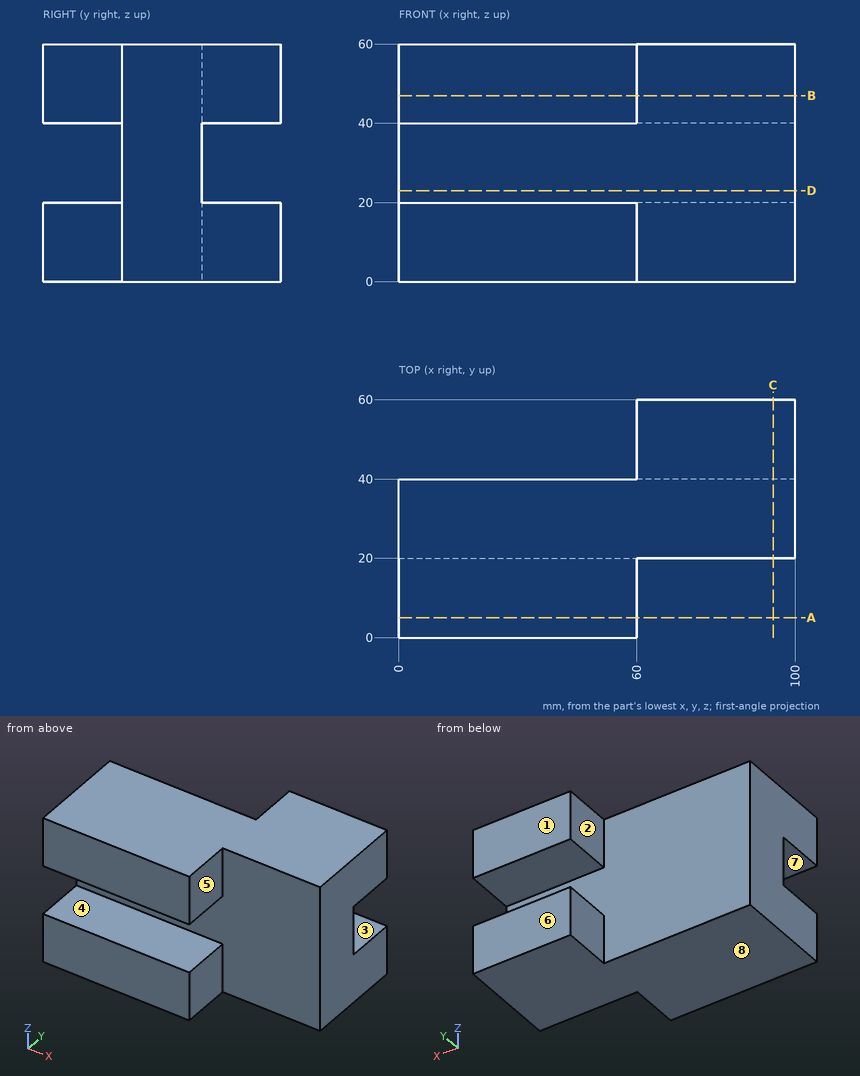
Input: dimensioned drawing with shaded views. Units: mm. Origin: part minimum x, y, z. A direction names the side the tool comes from. Coordinates: 2 decimals unless noted, no trailing zeros. Order: outer loops, then holes, each group sorted by start corner. A loop starts at its lowest first (then second) coordinate and runs counter-clockwise, first axis right, second up.
Item 1: Section query D-D (z = 23). Output: boundary loops of the cut face in (x, y), then the cut area to 3 significant figures.
Answer:
outline: (0, 20) - (100, 20) - (100, 40) - (0, 40) - close
area: 2,000 mm2
Item 2: Section query A-A (y = 5). Output: boundary loops of the cut face in (x, z).
Answer:
outline: (0, 0) - (60, 0) - (60, 20) - (0, 20) - close; (0, 40) - (60, 40) - (60, 60) - (0, 60) - close
Item 3: Material intervals for line 1 along Z through (x, y) = (78, 42.5); line 2 along X through (y, z) = (46.5, 5.5); line 3 along Y through (x, z) = (94.5, 53), sorted ascending.
Answer:
line 1: z = 0 to 20, 40 to 60
line 2: x = 60 to 100
line 3: y = 20 to 60
Item 4: Contact query for flat-ended pins moving along their axis: P1, Ø10, axis at x = 32, z = 25.5, coming from the -Y side; P2, Ø16, axis at y = 8, z = 14, coming from the +X side; P3, Ø6, axis at y = 48, z = 10.5, coming from the -X side. Output: stop coordinate, or through.
Answer:
P1: stops at y = 20
P2: stops at x = 60
P3: stops at x = 60
Item 5: Draft query along Z for the marked faces 6, 7 and 8. Return one class per face: released by +Z, released by -Z, zero draft, split by the parting line, or undercut.
Answer:
face 6: zero draft
face 7: undercut
face 8: released by -Z
Item 6: Section query B-B (z = 47). Output: boundary loops of the cut face in (x, y), then the cut area to 3 significant figures.
Answer:
outline: (0, 0) - (60, 0) - (60, 20) - (100, 20) - (100, 60) - (60, 60) - (60, 40) - (0, 40) - close
area: 4,000 mm2
Item 7: Access query for the marked faces 1, 2, 3, 4 and 5. Directions: +Z, -Z, +X, -X, +Y, -Y. A direction counts if a zero-diameter tool reaches every point of the face in a straight line with its end or side. Return the directions, or none.
Answer:
face 1: +Z, -Z, +X, -X, +Y
face 2: +Z, -Z, -X, +Y
face 3: +X, -X, +Y
face 4: +X, -X, -Y
face 5: +Z, -Z, +X, -Y
Item 8: Section query C-C (x = 94.5). Output: boundary loops of the cut face in (y, z).
Answer:
outline: (20, 0) - (60, 0) - (60, 20) - (40, 20) - (40, 40) - (60, 40) - (60, 60) - (20, 60) - close
